Work out the finished part from the listing and answer in its coordinate system (mm). Face numbers are marked on the shaded views. A direction names the side the tool comes from. Coordinates: 2 decimals unless noted, no trailing zeros. Order: outer loops, then holes, each group sorted by start corner. A loop starts at its lowest first (then second) coordinate and runs counter-clockwise, first axis right, second up. Notation, with made-up numbers: (-17, 5.5) -> (-1, 5.5) arc R18 ccw to (-1, 40.5) -> close; hole circle Ø7 at (0, 35.5). An arc over 180 degrees is marked (long way). Write item = value, one per line. Start each with the question number.
Q1. The part is cut by section A-A, the plane y = 22. Determine the outline of the cut face in (x, z) (3 decimals).
Q2. Straight lines are drawn through the part: L1, parallel to X at y = 28, z = -14; L2, parallel to Z at x = -6, y = -25 (3 decimals); L3, parallel to Y at x = -12.5, z = -15. For each, find the intervals that lie inside material, in ascending order. Write a range as from..to.
Q3. For a pull along Z with two mould halves and no side action, classify the marked faces 3, 4 and 5 as +Z half, -Z half, draft (parallel to the pull), parting line (faces both ways), or undercut.
Q4. A flat-ended cylindrical pin translates along its axis: pin 1 (6 mm diameter, centred on x = -9.5, z = 14, fed in from +Y). Find the tip coordinate at first contact, or state that the pin passes through.
Q5. The part is cut by section B-B, the plane z = -28. Determine the outline of the cut face in (x, y).
Q6. Which of the six approach directions +Z, -Z, +X, -X, +Y, -Y give full straight-line access (tool end or side, diameter ignored) to the marked faces 1 and 2?
```python
from build123d import *

# Parameters (mm, degrees)
SKETCH1_W           = 26.162
SKETCH1_H           = 76.2
BOSS_EXTRUDE1_DEPTH = 38.1
SKETCH2_W           = 19.812
SKETCH2_H           = 69.85
CUT_EXTRUDE1_DEPTH  = 73.025
CHAMFER1_SIZE       = 4.7625
SKETCH3_W           = 6.35
SKETCH3_H           = 0.7874
BOSS_EXTRUDE2_DEPTH = 1.27
FILLET1_R           = 2.54
FILLET2_R           = 2.54


with BuildPart() as part:
    # Sketch1 → Boss-Extrude1 (new, symmetric)
    with BuildSketch(Plane.XY):
        with Locations((-6.755190476, 6.28952381)):
            Rectangle(SKETCH1_W, SKETCH1_H)
    extrude(amount=BOSS_EXTRUDE1_DEPTH, both=True)

    # Sketch2 → Cut-Extrude1 (cut)
    with BuildSketch(Plane(origin=(0, 44.38952381, 0), x_dir=(1, 0, 0), z_dir=(0, 1, 0))):
        with Locations((-6.755190476, 0)):
            Rectangle(SKETCH2_W, SKETCH2_H)
    extrude(amount=-CUT_EXTRUDE1_DEPTH, mode=Mode.SUBTRACT)

    # Chamfer1
    chamfer1_edges = [part.edges().sort_by_distance(p)[0] for p in [
        (-6.755190476, -31.81047619, 38.1),
        (-6.755190476, -31.81047619, -38.1),
        (6.325809524, -31.81047619, 0),
        (-19.836190476, -31.81047619, 0),
    ]]
    chamfer(chamfer1_edges, length=CHAMFER1_SIZE)

    # Sketch3 → Boss-Extrude2 (add)
    with BuildSketch(Plane(origin=(0, 0, 34.925), x_dir=(-1, 0, 0), z_dir=(0, 0, -1))):
        with Locations((6.755190476, 43.99582381)):
            Rectangle(SKETCH3_W, SKETCH3_H)
    extrude(amount=BOSS_EXTRUDE2_DEPTH)

    # Fillet1
    fillet1_edges = [part.edges().sort_by_distance(p)[0] for p in [
        (6.325809524, 8.67077381, -38.1),
        (6.325809524, 8.67077381, 38.1),
        (-19.836190476, 8.67077381, -38.1),
        (-19.836190476, 8.67077381, 38.1),
    ]]
    fillet(fillet1_edges, radius=FILLET1_R)

    # Fillet2
    # the kernel refuses this fillet: 2.54 mm, written as the material it takes off along each edge
    with BuildSketch(Plane(origin=(-3.580190476, 49.888785124, 33.655), x_dir=(0, 0, 1), z_dir=(0, -1, 0))) as fillet2_piece_1:
        with BuildLine():
            CenterArc((2.54, 2.199704526), FILLET2_R, 180, 60)
            Line((0, 2.199704526), (-0.0508, 2.199704526))
            Line((-0.0508, 2.199704526), (-0.0508, 0))
            Line((-0.0508, 0), (0, -0.0508))
            ThreePointArc((0, -0.0508), (0.635, -0.0508), (1.2446, -0.043994091))
            Line((1.2446, -0.043994091), (1.27, 0))
        make_face()
    extrude(amount=11.785922628, mode=Mode.SUBTRACT)
    with BuildSketch(Plane(origin=(-9.930190476, 38.102862495, 33.655), x_dir=(1, 0, 0), z_dir=(0, 1, 0))) as fillet2_piece_2:
        with BuildLine():
            CenterArc((2.199704526, -2.54), FILLET2_R, 90, 60)
            Line((0, -1.27), (-0.043994091, -1.2446))
            ThreePointArc((-0.043994091, -1.2446), (-0.0508, -0.635), (-0.0508, 0))
            Line((-0.0508, 0), (0, 0.0508))
            Line((0, 0.0508), (2.199704526, 0.0508))
            Line((2.199704526, 0.0508), (2.199704526, 0))
        make_face()
    extrude(amount=11.785922628, mode=Mode.SUBTRACT)


solid = part.part
```
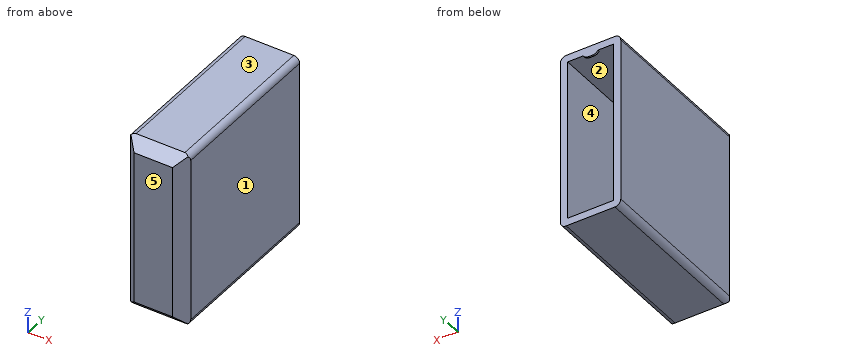
Model answer:
q1.outline = (-19.836, -35.56) arc R2.54 ccw to (-17.296, -38.1) -> (3.786, -38.1) arc R2.54 ccw to (6.326, -35.56) -> (6.326, 35.56) arc R2.54 ccw to (3.786, 38.1) -> (-17.296, 38.1) arc R2.54 ccw to (-19.836, 35.56) -> close; hole (-16.661, -34.925) -> (3.151, -34.925) -> (3.151, 34.925) -> (-16.661, 34.925) -> close
q2.L1 = -19.84..-16.66, 3.15..6.33
q2.L2 = -38.1..-34.925, 34.925..38.1
q2.L3 = -31.81..-28.64
q3.face_3 = +Z half
q3.face_4 = undercut
q3.face_5 = draft
q4.pin_1 = -28.64
q5.outline = (-19.84, -27.05) -> (-15.07, -31.81) -> (1.56, -31.81) -> (6.33, -27.05) -> (6.33, 44.39) -> (3.15, 44.39) -> (3.15, -28.64) -> (-16.66, -28.64) -> (-16.66, 44.39) -> (-19.84, 44.39) -> close
q6.face_1 = +Z, -Z, +X, +Y, -Y
q6.face_2 = none
